```python
from build123d import *

# Parameters (mm, degrees)
SKETCH1_R           = 12.5
BOSS_EXTRUDE1_DEPTH = 138.5
SKETCH2_R           = 13.5
BOSS_EXTRUDE2_DEPTH = 37
BOSS_EXTRUDE3_START = 28
SKETCH3_R           = 13.5
BOSS_EXTRUDE3_DEPTH = 28
CUT_EXTRUDE1_START  = -21
CUT_EXTRUDE1_DEPTH  = 21
SKETCH5_R           = 4
CUT_EXTRUDE2_DEPTH  = 178.32667594
CUT_EXTRUDE4_START  = -21
CUT_EXTRUDE4_DEPTH  = 21
CUT_EXTRUDE5_DEPTH  = 20
SKETCH8_OUTSIDE_W   = 70.41
SKETCH8_OUTSIDE_H   = 70.41
SKETCH8_OUTSIDE_R   = 11.25
CUT_EXTRUDE6_DEPTH  = 12
SKETCH10_R          = 4.5
CUT_EXTRUDE7_DEPTH  = 12
SKETCH11_R          = 4
CUT_EXTRUDE8_DEPTH  = 12


with BuildPart() as part:
    # Sketch1 → Boss-Extrude1 (new body)
    with BuildSketch(Plane.XY):
        Circle(SKETCH1_R)
    extrude(amount=BOSS_EXTRUDE1_DEPTH)

    # Sketch2 → Boss-Extrude2 (add)
    with BuildSketch(Plane.XY.offset(138.5)):
        Circle(SKETCH2_R)
    extrude(amount=BOSS_EXTRUDE2_DEPTH)

    # Sketch3 → Boss-Extrude3 (add)
    with BuildSketch(Plane(origin=(0, 0, 0), x_dir=(-1, 0, 0), z_dir=(0, 0, -1)).offset(BOSS_EXTRUDE3_START)):
        with Locations(Location((0, 0, 0), (0, 0, 180))):
            Circle(SKETCH3_R)
    extrude(amount=-BOSS_EXTRUDE3_DEPTH)

    # Sketch4 → Cut-Extrude1 (cut)
    with BuildSketch(Plane.XY.offset(175.5).offset(CUT_EXTRUDE1_START)):
        with BuildLine():
            Line((-8, 10.874281585), (-8, -10.874281585))
            ThreePointArc((-8, -10.874281585), (-13.5, 0), (-8, 10.874281585))
        make_face()
        with BuildLine():
            Line((8, 10.874281585), (8, -10.874281585))
            ThreePointArc((8, -10.874281585), (13.5, 0), (8, 10.874281585))
        make_face()
    extrude(amount=CUT_EXTRUDE1_DEPTH, mode=Mode.SUBTRACT)

    # Sketch5 → Cut-Extrude2 (cut, through all)
    with BuildSketch(Plane.ZY.offset(8)):
        with Locations((166.5, 0)):
            Circle(SKETCH5_R)
    extrude(amount=-CUT_EXTRUDE2_DEPTH, mode=Mode.SUBTRACT)

    # Sketch6 → Cut-Extrude4 (cut)
    with BuildSketch(Plane.XY.offset(175.5).offset(CUT_EXTRUDE4_START)):
        with BuildLine():
            Line((8, 10.874281585), (8, 7.549834435))
            ThreePointArc((8, 7.549834435), (0, 11), (-8, 7.549834435))
            Line((-8, 7.549834435), (-8, 10.874281585))
            ThreePointArc((-8, 10.874281585), (0, 13.5), (8, 10.874281585))
        make_face()
        with BuildLine():
            Line((-8, -10.874281585), (-8, -7.549834435))
            ThreePointArc((-8, -7.549834435), (0, -11), (8, -7.549834435))
            Line((8, -7.549834435), (8, -10.874281585))
            ThreePointArc((8, -10.874281585), (0, -13.5), (-8, -10.874281585))
        make_face()
    extrude(amount=CUT_EXTRUDE4_DEPTH, mode=Mode.SUBTRACT)

    # Sketch7 → Cut-Extrude5 (cut)
    with BuildSketch(Plane(origin=(0, 0, -28), x_dir=(-1, 0, 0), z_dir=(0, 0, -1))):
        with BuildLine():
            Line((-12, 6.184658438), (-12, -6.184658438))
            ThreePointArc((-12, -6.184658438), (-13.5, 0), (-12, 6.184658438))
        make_face()
        with BuildLine():
            Line((12, 6.184658438), (12, -6.184658438))
            ThreePointArc((12, -6.184658438), (13.5, 0), (12, 6.184658438))
        make_face()
    extrude(amount=-CUT_EXTRUDE5_DEPTH, mode=Mode.SUBTRACT)

    # Sketch8 outside → Cut-Extrude6 (cut)
    with BuildSketch(Plane(origin=(0, 0, -28), x_dir=(-1, 0, 0), z_dir=(0, 0, -1))):
        Rectangle(SKETCH8_OUTSIDE_W, SKETCH8_OUTSIDE_H)
        Circle(SKETCH8_OUTSIDE_R, mode=Mode.SUBTRACT)
    extrude(amount=-CUT_EXTRUDE6_DEPTH, mode=Mode.SUBTRACT)

    # Sketch10 → Cut-Extrude7 (cut)
    with BuildSketch(Plane(origin=(0, 15, 0), x_dir=(-1, 0, 0), z_dir=(0, 1, 0))):
        with Locations(Location((0, 146.266828113, 0), (0, 0, 90))):
            Circle(SKETCH10_R)
        with Locations(Location((0, -8.332143665, 0), (0, 0, 90))):
            Circle(SKETCH10_R)
    extrude(amount=-CUT_EXTRUDE7_DEPTH, mode=Mode.SUBTRACT)

    # Sketch11 → Cut-Extrude8 (cut)
    with BuildSketch(Plane(origin=(0, 0, -28), x_dir=(-1, 0, 0), z_dir=(0, 0, -1))):
        Circle(SKETCH11_R)
    extrude(amount=-CUT_EXTRUDE8_DEPTH, mode=Mode.SUBTRACT)


solid = part.part
```
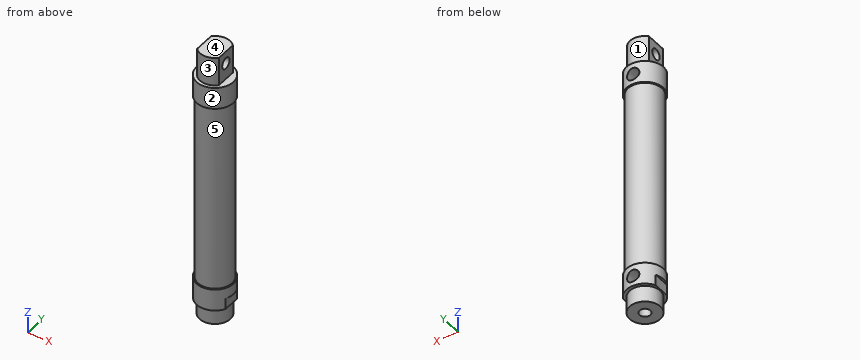
Design review of the part built by this model. Coordinates are the model's own, in mm. Face numbers are marked on the shaded views. A direction names the side the tool comes from. Give positions to 0.01 mm unless a question says otherwise; leave off trailing zeros. Order: outer loops, then holes, each group sorted by start corner. A loop starts at its lowest first (then second) coordinate and runs counter-clockwise, first axis right, second up. Notation, with made-up numbers: (70.5, 74.25) -> (117.5, 74.25) arc R38 cw to (117.5, 113.25) -> close; hole circle Ø2 at (-23, -21). An arc over 180 degrees is marked (long way). Write each question's results on one line, items separated by ' | '. Start each with the question number.
Q1. Add section A-A on z = 166.5. Give the boundary of the cut face in (x, y), and give its area (3 significant figures).
Q2. Machinability: for the marked faces 1 and 2, which of the approach directions +Z, -Z, +X, -X, +Y, -Y give a long, thin tool a straight path to every point of the face, cutting with its end or side? Answer none if there is none.
Q3. Mouldability with a two-part tool opening along Z and no side actions: class the marked faces 3, 4 and 5 as +Z half, -Z half, draft (parallel to the pull), parting line (faces both ways), or undercut.
Q4. For pin 1 (7.5 mm diameter, centred on y = 3, z = 165.5, fed in from +X); pin 2 (10 mm diameter, centred on y = 6.5, z = -1, fed in from +X); pin 3 (4 mm diameter, centred on x = -0.5, z = 71, fed in from -Y), all flat-tipped, find the tip position at first contact; note any pin that passes through.
Q5. Wall thickness on L1, parallel to Z at x = 0, y = 7.75; L2, parallel to Y at x = 0, z = -22.5; L3, parallel to Z at x = -10.5, y = 2.5: over which ranges is each line inside the solid? List them lowest first. Write a range as from..to.
Q6. Add section D-D on z = 130. Give the boundary of the cut face in (x, y).
Found:
1) outline: (-8, -7.55) arc R11 ccw to (8, -7.55) -> (8, -4) -> (-8, -4) -> close; (-8, 4) -> (8, 4) -> (8, 7.55) arc R11 ccw to (-8, 7.55) -> close | area: 190 mm2
2) face 1: +Z, +Y | face 2: +Z, -Z
3) face 3: draft | face 4: +Z half | face 5: undercut
4) pin 1: stops at x = 8 | pin 2: stops at x = 13.42 | pin 3: stops at y = -12.5
5) L1: z = -28..-12.83, -3.83..141.77, 150.77..175.5 | L2: y = -11.25..-4, 4..11.25 | L3: z = -28..154.5
6) outline: circle Ø25 at (0, 0)
